Drawing for the job (mm, zero at the part's lowest x, y, z). A direction names the side the tool comes from. Round coordinates to 2 decimals unless told otherwise and drop trailing zeros. Write each loop counter-clockwise with the first axis right and the second up, starting at its lowest first coordinate (ties: lowest second). Pieces come first, ordered by that corner, then holes. Notation, with made-up numbers: M 64.5,19 L 116.5,19 A28 cw 116.5,37 Z; hole C 4,21 d4. An arc over 180 degrees is marked long. Use a Markdown table: item, result.
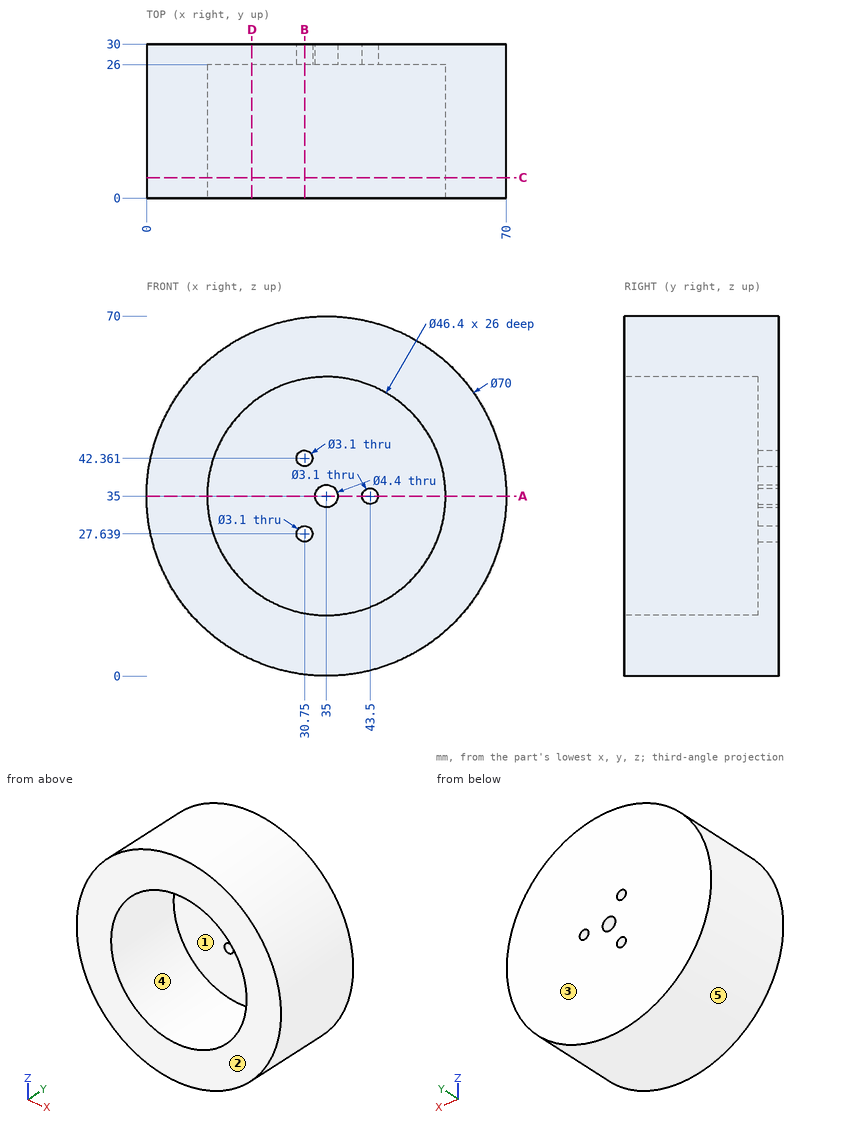
Q1. Drill centre lines: L1, parallel to Z at x = 30.75, y = 28.65; L2, parallel to Z at x = 35, y = 29.25; L3, parallel to Z at x = 35, y = 6. Where is each one in solid material? Low to high.
Response values:
| item | result |
|---|---|
| L1 | z = 0.26 to 26.09, 29.19 to 40.81, 43.91 to 69.74 |
| L2 | z = 0 to 32.8, 37.2 to 70 |
| L3 | z = 0 to 11.8, 58.2 to 70 |
Q2. Cut at D-D on x = 20.5. Give the cut face in (y, z) (1 decimal).
Response values:
| item | result |
|---|---|
| outline | M 0,3.1 L 30,3.1 L 30,66.9 L 0,66.9 L 0,53.1 L 26,53.1 L 26,16.9 L 0,16.9 Z |
Q3. Cut at C-C on y = 4. Give the cut face in (x, z).
Response values:
| item | result |
|---|---|
| outline | C 35,35 d70; hole C 35,35 d46.4 |
Q4. Which spindle directions (+Z, -Z, +X, -X, +Y, -Y) get a long thin tool onto all of the face, cutting with end or side? Do the marked faces 1 and 2. Say none if no direction does.
Response values:
| item | result |
|---|---|
| face 1 | -Y |
| face 2 | +Z, -Z, +X, -X, -Y |
Q5. Two-plate mould, pull along X, no slides. Class the marked faces 3, 4 and 5: +X half, -X half, draft (parallel to the pull), parting line (faces both ways), or undercut.
Response values:
| item | result |
|---|---|
| face 3 | draft |
| face 4 | undercut |
| face 5 | parting line |
Q6. Cut at B-B on x = 30.75. Give the cut face in (y, z), and give its area (3 significant figures).
Response values:
| item | result |
|---|---|
| outline | M 0,0.26 L 30,0.26 L 30,26.09 L 26,26.09 L 26,12.19 L 0,12.19 Z; M 0,57.81 L 26,57.81 L 26,43.91 L 30,43.91 L 30,69.74 L 0,69.74 Z; M 26,29.19 L 30,29.19 L 30,40.81 L 26,40.81 Z |
| area | 874 mm2 |
Q7. Drop flat-ended pins along their axis: P1, Ø4, axis at y = 16.5, z = 19, coming from the -X side; P2, Ø10, axis at y = 19.5, z = 52, coming from the +X side; P3, Ø3, axis at y = 15.5, z = 62.5, coming from the +X side. Give the stop position or say it passes through.
Response values:
| item | result |
|---|---|
| P1 | stops at x = 2.92 |
| P2 | stops at x = 67.88 |
| P3 | stops at x = 58.43 |
Q8. Cut at A-A on z = 35. Give the cut face in (x, y).
Response values:
| item | result |
|---|---|
| outline | M 0,0 L 11.8,0 L 11.8,26 L 32.8,26 L 32.8,30 L 0,30 Z; M 37.2,26 L 41.95,26 L 41.95,30 L 37.2,30 Z; M 45.05,26 L 58.2,26 L 58.2,0 L 70,0 L 70,30 L 45.05,30 Z |
